Here's the drawing with two shaded views (mm, measured from the low corner). I have some questions. Coordinates: 2 decimals unless noted, no trailing zeros. Write each loop counter-clockwise with the first axis right and the second up, starting at its lowest first coordinate (ties: lowest second). Pieces come first, ordered by that corner, then holes.
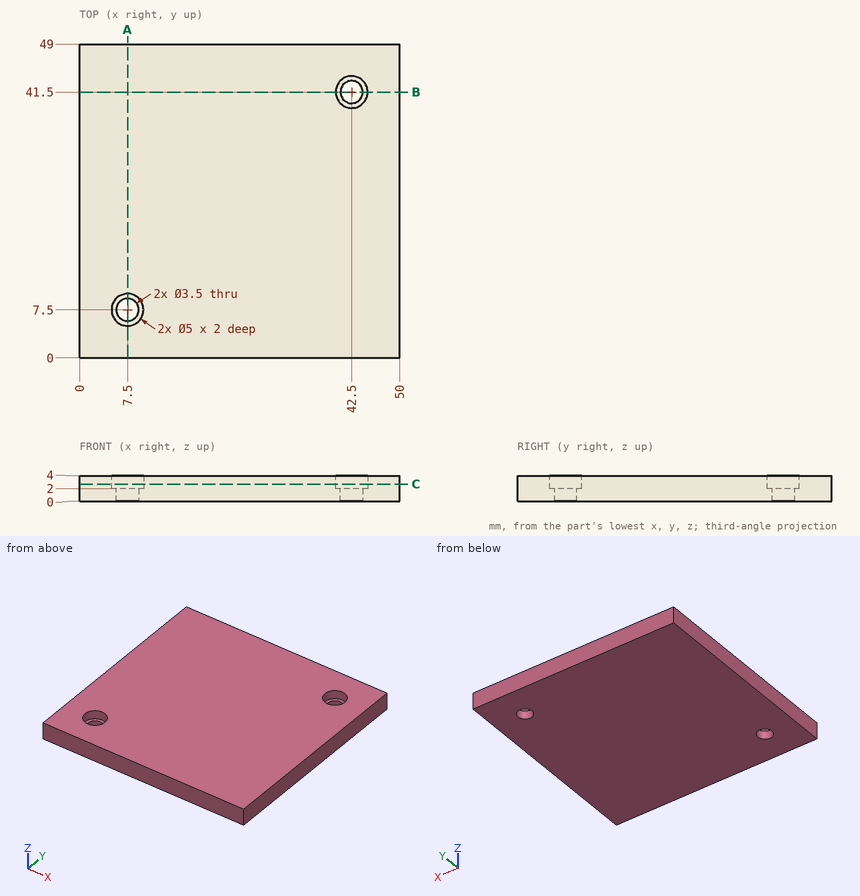
1. I want a section at B-B on y = 41.5. Please give me the cut outline in (x, z).
Verdict:
outline: (0, 0) - (40.75, 0) - (40.75, 2) - (40, 2) - (40, 4) - (0, 4) - close; (44.25, 0) - (50, 0) - (50, 4) - (45, 4) - (45, 2) - (44.25, 2) - close
2. Please list where these lines run through material, in increasing order: line 1 along Y through (x, z) = (42.5, 2.85); line 2 along Y through (x, z) = (7.5, 2.7); line 3 along X through (y, z) = (40, 1.2).
Verdict:
line 1: y = 0 to 39, 44 to 49
line 2: y = 0 to 5, 10 to 49
line 3: x = 0 to 41.6, 43.4 to 50
3. I want a section at A-A on x = 7.5. Please give me the cut outline in (y, z), plus the area to 3 significant figures.
Verdict:
outline: (0, 0) - (5.75, 0) - (5.75, 2) - (5, 2) - (5, 4) - (0, 4) - close; (9.25, 0) - (49, 0) - (49, 4) - (10, 4) - (10, 2) - (9.25, 2) - close
area: 179 mm2
4. I want a section at C-C on z = 2.7. Please give me the cut outline in (x, y).
Verdict:
outline: (0, 0) - (50, 0) - (50, 49) - (0, 49) - close; hole circle Ø5 at (7.5, 7.5); hole circle Ø5 at (42.5, 41.5)
5. For pin 1 (4 mm diameter, centred on x = 42.5, y = 41.5, fed in from +Z); pin 2 (3 mm diameter, centred on x = 42.5, y = 41.5, fed in from +Z), each with a flat end and sliding along its axis, tell me the tip position at first contact or that it passes through.
Verdict:
pin 1: stops at z = 2
pin 2: passes through
